Geometry check sheet. Reference: the model listing, model coordinates, mm. Round coordinates to 2 decimals unless told otherwise and drop trailing zeros. Write each loop counter-clockwise with the first axis right and the second up, starting at its lowest first coordinate (ties: lowest second). Pieces come first, ordered by that corner, then holes. Notation, with made-up numbers: (68, 17.5) -> (93, 17.5) arc R23 ccw to (93, 45.5) -> close; hole circle Ø1 at (44.5, -9.75). An arc over 180 degrees is marked (long way). Use a Markdown table: item, result.
```python
from build123d import *

# Parameters (mm, degrees)
SKETCH_1_R      = 1.5
EXTRUDE_1_DEPTH = 5


with BuildPart() as part:
    # 草图1 → 凸台-拉伸1 (new body)
    with BuildSketch(Plane.XY):
        Polygon((96.244173447, 49.032986466), (-3.755826553, 49.032986466), (-68.755826553, 49.032986466), (-76.755820543, 41.032992475), (-76.755820543, -33.967007525), (-68.755826553, -41.967013534), (96.244173447, -41.967013534), (104.244173447, -33.967013534), (104.244173447, 41.032986466), align=None)
        with Locations((-68.755826553, -33.967007525)):
            Circle(SKETCH_1_R, mode=Mode.SUBTRACT)
        with Locations((-3.755826553, -33.967013534)):
            Circle(SKETCH_1_R, mode=Mode.SUBTRACT)
        with Locations((-3.755826553, -10.967013534)):
            Circle(SKETCH_1_R, mode=Mode.SUBTRACT)
        with Locations((96.244173447, -33.967013534)):
            Circle(SKETCH_1_R, mode=Mode.SUBTRACT)
        Polygon((-64.826894365, -28.310159285), (-64.826894365, 35.376132216), (-10.826894365, 35.376132216), (-10.826894365, 28.305064404), (-10.826894365, -28.310159285), align=None, mode=Mode.SUBTRACT)
        with Locations((-3.755826553, 6.032986466)):
            Circle(SKETCH_1_R, mode=Mode.SUBTRACT)
        with Locations((-68.755826553, 41.032992475)):
            Circle(SKETCH_1_R, mode=Mode.SUBTRACT)
        with Locations((-3.755826553, 41.032986466)):
            Circle(SKETCH_1_R, mode=Mode.SUBTRACT)
        Polygon((90.587319198, -28.310159285), (3.315241259, -28.310159285), (3.315241259, 28.305064404), (3.315241259, 35.376132216), (90.587319198, 35.376132216), align=None, mode=Mode.SUBTRACT)
        with Locations((96.244173447, 41.032986466)):
            Circle(SKETCH_1_R, mode=Mode.SUBTRACT)
    extrude(amount=EXTRUDE_1_DEPTH)


solid = part.part
```
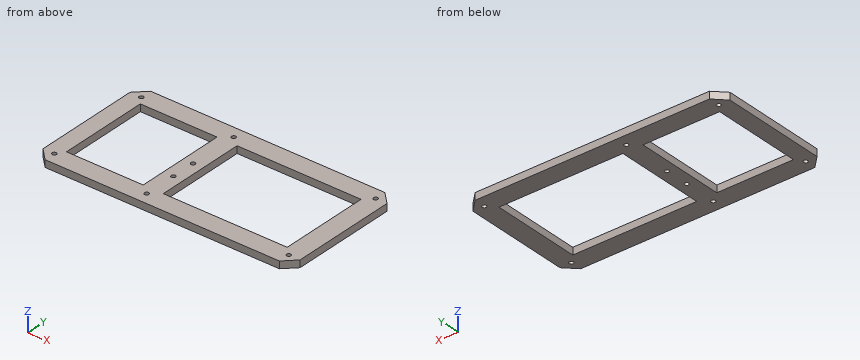
(1) Section check A-A on x = 77. Record the cut outline in (y, z), plus the area to 3 significant figures.
A:
| item | result |
|---|---|
| outline | (-41.97, 0) -> (-28.31, 0) -> (-28.31, 5) -> (-41.97, 5) -> close; (35.38, 0) -> (49.03, 0) -> (49.03, 5) -> (35.38, 5) -> close |
| area | 137 mm2 |
(2) Thickness scan on line 1 (X direction, y = -17.5, z = 4.75); line 2 (Y direction, x = -27.5, z = 2.8); line 3 (X direction, y = 6, z = 1.15). Record the ranges inside material, lowest first.
A:
| item | result |
|---|---|
| line 1 | x = -76.76 to -64.83, -10.83 to 3.32, 90.59 to 104.24 |
| line 2 | y = -41.97 to -28.31, 35.38 to 49.03 |
| line 3 | x = -76.76 to -64.83, -10.83 to -5.26, -2.26 to 3.32, 90.59 to 104.24 |
(3) Section check B-B on y = -14.5. Record the cut outline in (x, z).
A:
| item | result |
|---|---|
| outline | (-76.76, 0) -> (-64.83, 0) -> (-64.83, 5) -> (-76.76, 5) -> close; (-10.83, 0) -> (3.32, 0) -> (3.32, 5) -> (-10.83, 5) -> close; (90.59, 0) -> (104.24, 0) -> (104.24, 5) -> (90.59, 5) -> close |
(4) Section check C-C on z = 1.55. State how many separate pieces and enclosed holes the cut face has, plus the area to 3 significant figures.
A:
| item | result |
|---|---|
| separate pieces | 1 |
| enclosed holes | 10 |
| area | 7,290 mm2 |
